For this review, take the finished solid that the model builds, in its own axes (mm). A direction names the side the tool comes from. Give positions to 0.01 mm unless a question says otherwise; leave off trailing zeros. Write each loop counter-clockwise with the first axis right and the second up, starting at its lowest first coordinate (ties: lowest second). Pieces come first, ordered by that corner, then holes. Notation, with made-up numbers: M 29,88 L 54,88 A31 cw 54,112 Z; hole C 63,27 d4. An arc over 180 degrees is marked long. One line per item, written item: value. Start each with the question number.
Item 1: To check wall thickness, follow probe 1 along X at (y, z) = (23.5, -0.8) (3 decimals); probe 2 along X at (y, z) = (14.5, -2) (3 decimals); probe 3 along Y at (x, z) = (5.75, -1.25). State the ranges of each line that lie inside material, in increasing order.
Item 2: Consider section D-D, the plane y = 3.5. Write out the cut boundary in (x, z).
Item 3: Tool access review of faces 4 (the face through (4, 21, -2.2)), 5 (the face through (8.059, 13.828, -1.597)), 6 (the face through (11.525, 19, -1)): name each direction out of +Z, -Z, +X, -X, +Y, -Y from which nothing blocks a thin tool from reaching the whole face with its end or side.
Item 4: Consider section C-C, the plane y = 25. Write out the cut boundary in (x, z) (3 decimals), and give its area (3 significant figures).
Item 5: Mouldability with a two-part tool opening along X and no side actions: class faces 1 (the face through (8, 40.5, -1)), 2 (the face through (8, 11.362, -1)), 3 (the face through (0, 20, -1)) as released by +X, released by -X, zero draft, split by the parting line, or undercut.
Item 6: Clearance check with flat-ended pins moving along their axes: pin 1 Ø0.6 at (y, z) = (15.5, 0.5) entering from -X (3 decimals); pin 2 Ø0.5 at (x, z) = (7.5, 0.5) entering from +Y; pin 3 Ø1.5 at (x, y) = (5, 6.5) entering from +Z. State where each tip first meets the part, or that it passes through.
```python
from build123d import *

# Parameters (mm, degrees)
F0_W         = 16.2
F0_H         = 40.5
F1_DEPTH     = 2.2
F0_W_2       = 5.85
F0_H_2       = 15.625
F0_W_3       = 5.55
F0_H_3       = 2.375
F2_DEPTH     = 1.8
F3_DEPTH     = 0.6
F4_T1_DEPTH  = 5.85
F4_T6_DEPTH  = 18.8484687937
F4_T11_DEPTH = 5.85
F4_T16_DEPTH = 18.8484687937
F5_SIZE      = 0.39999


# Not quite as in the source:
# - a fillet or chamfer that OpenCascade refuses, or shapes differently, is made with other operations: its cross-section is extruded or revolved along the edge and cut away or added
# - a fillet or chamfer is up to 0.001 mm smaller than in the source, because OpenCascade refuses the exact size


with BuildPart() as f1:
    # F0 (on Top) → F1 (new body)
    with BuildSketch(Plane.XY):
        with Locations((8.1, 20.25)):
            Rectangle(F0_W, F0_H)
        with BuildLine():
            Line((11.275, 10.8625), (4.925, 10.8625))
            ThreePointArc((4.925, 10.8625), (4.7482233047, 10.9357233047), (4.675, 11.1125))
            Line((4.675, 11.1125), (4.675, 26.9875))
            ThreePointArc((4.675, 26.9875), (4.925, 27.2375), (5.175, 26.9875))
            Line((5.175, 26.9875), (11.025, 26.9875))
            ThreePointArc((11.025, 26.9875), (11.275, 27.2375), (11.525, 26.9875))
            Line((11.525, 26.9875), (11.525, 11.1125))
            ThreePointArc((11.525, 11.1125), (11.4517766953, 10.9357233047), (11.275, 10.8625))
        make_face(mode=Mode.SUBTRACT)
    extrude(amount=-F1_DEPTH)

    # F0 (on Top) → F2 (join)
    with BuildSketch(Plane.XY):
        with Locations((8.1, 19.175)):
            Rectangle(F0_W_2, F0_H_2)
        with Locations((8.1, 15.875)):
            Rectangle(F0_W_3, F0_H_3, mode=Mode.SUBTRACT)
        with Locations((8.1, 15.875)):
            Rectangle(F0_W_3, F0_H_3)
    extrude(amount=-F2_DEPTH)

    # F0 (on Top) → F3 (join)
    with BuildSketch(Plane.XY):
        with Locations((8.1, 15.875)):
            Rectangle(F0_W_3, F0_H_3)
    extrude(amount=F3_DEPTH)

    # F4: chamfer of 5 x 0.4 on 2 edges, made by hand

    # F4_s2 → F4_t1 (cut)
    with BuildSketch(Plane.YZ.offset(5.175)):
        Polygon((11.3625, -1.4), (16.3625, -1.8), (11.3625, -1.8), align=None)
    extrude(amount=F4_T1_DEPTH, mode=Mode.SUBTRACT)


with BuildPart() as f4_tool4:
    # F4_s5 → F4_t6 (new body)
    with BuildSketch(Plane.YZ.offset(5.175)):
        Polygon((16.3625, 0), (11.3625, -0.4), (11.3625, 0), align=None)
    extrude(amount=F4_T6_DEPTH)

    split(bisect_by=Plane.YZ.offset(5.325), keep=Keep.BOTTOM)


with BuildPart() as f1_1:
    add(f1.part)

    # F4_t3: cut F4_tool4
    add(f4_tool4.part, mode=Mode.SUBTRACT)


with BuildPart() as f4_tool9:
    # F4_s10 → F4_t11 (new body)
    with BuildSketch(Plane.YZ.offset(5.175)):
        Polygon((16.3625, 0), (11.3625, -0.4), (11.3625, 0), align=None)
    extrude(amount=F4_T11_DEPTH)

    split(bisect_by=Plane.XZ.offset(-14.6875), keep=Keep.TOP)


with BuildPart() as f1_2:
    add(f1_1.part)

    # F4_t8: cut F4_tool9
    add(f4_tool9.part, mode=Mode.SUBTRACT)


with BuildPart() as f4_tool14:
    # F4_s15 → F4_t16 (new body)
    with BuildSketch(Plane.YZ.offset(-7.8234687937)):
        Polygon((16.3625, 0), (11.3625, -0.4), (11.3625, 0), align=None)
    extrude(amount=F4_T16_DEPTH)

    split(bisect_by=Plane.YZ.offset(10.875), keep=Keep.TOP)


with BuildPart() as f1_3:
    add(f1_2.part)

    # F4_t13: cut F4_tool14
    add(f4_tool14.part, mode=Mode.SUBTRACT)

    # F5 (size 0.4 in the source; OpenCascade refuses exactly that, so slightly less here)
    f5_edges = [f1_3.edges().sort_by_distance(p)[0] for p in [
        (8.1, 14.6875, 0.6),
        (8.1, 26.9875, -1.8),
    ]]
    chamfer(f5_edges, length=F5_SIZE)


solid = f1_3.part
```
Model answer:
1. probe 1: x = 0 to 4.675, 5.175 to 11.025, 11.525 to 16.2
1. probe 2: x = 0 to 4.675, 11.525 to 16.2
1. probe 3: y = 0 to 10.86, 11.36 to 40.5
2. outline: M 0,-2.2 L 16.2,-2.2 L 16.2,0 L 0,0 Z
3. face 4: -Z, +X, -X, +Y, -Y
3. face 5: -Z
3. face 6: +Z, -Z
4. outline: M 0,-2.2 L 4.675,-2.2 L 4.675,0 L 0,0 Z; M 5.175,-1.8 L 11.025,-1.8 L 11.025,0 L 5.175,0 Z; M 11.525,-2.2 L 16.2,-2.2 L 16.2,0 L 11.525,0 Z
4. area: 31.1 mm2
5. face 1: zero draft
5. face 2: undercut
5. face 3: released by -X
6. pin 1: stops at x = 5.325
6. pin 2: stops at y = 17.06
6. pin 3: stops at z = 0
